Read the model definition and answer for the solid it produces. Units are mm, in the model's axes. Coordinates: 2 decimals unless noted, no trailing zeros. Loops run counter-clockwise (first coordinate to the right, second up) from the corner with the lowest first, then second, coordinate; pieces in that order, holes last.
Q1. Section C-C (x = -10.5) is taken. Give the vertices of the cut face in (y, z).
Q2. Section B-B (y = 23.5) is taken. Give the vertices of the cut face in (x, z), then the cut area to 3 significant figures.
Q3. Straight lines are drawn through the part: line 1 (Y direction, x = -3, z = -0.3); line 2 (X direction, y = 18.5, z = -0.4); line 3 (X direction, y = 9.5, z = -0.95). For each, find the intervals that lie inside material, in ascending order.
Q4. A flat-ended cylindrical pin translates along its axis: P1, Ø0.6, axis at x = -15, z = -0.5, coming from the +Y side. Find the tip coordinate at first contact, or state that the pin passes through.
Q5. Section A-A (z = -1) is taken. Give the vertices of the cut face in (x, y).
from build123d import *

# Parameters (mm, degrees)
SM_BASE_FLANGE_1_DEPTH = 1.2


# Sheet-metal steps are written as plain solids
with BuildPart() as part:
    # Sketch 1 → 基体-法兰1 (new body)
    with BuildSketch(Plane.XY):
        with BuildLine():
            Line((0, 0), (-26, 0))
            ThreePointArc((-26, 0), (-29, 3), (-26, 6))
            ThreePointArc((-26, 6), (-23, 9), (-26, 12))
            ThreePointArc((-26, 12), (-29, 15), (-26, 18))
            Line((-26, 18), (0, 18))
            Line((0, 18), (11.606526016, 25.828700649))
            ThreePointArc((11.606526016, 25.828700649), (15.771217444, 25.019166641), (14.961683437, 20.854475213))
            ThreePointArc((14.961683437, 20.854475213), (14.152149429, 16.689783785), (18.316840857, 15.880249778))
            ThreePointArc((18.316840857, 15.880249778), (22.481532285, 15.070715771), (21.671998278, 10.906024343))
            Line((21.671998278, 10.906024343), (5.503152266, 0))
            Line((5.503152266, 0), (0, 0))
        make_face()
    extrude(amount=-SM_BASE_FLANGE_1_DEPTH)


solid = part.part
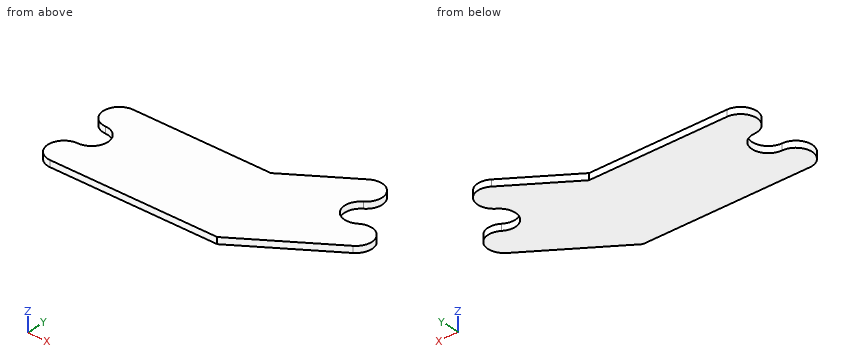
Numbers:
1. outline: (0, -1.2) - (18, -1.2) - (18, 0) - (0, 0) - close
2. outline: (8.15, -1.2) - (16.28, -1.2) - (16.28, 0) - (8.15, 0) - close
2. area: 9.75 mm2
3. line 1: y = 0 to 18
3. line 2: x = 0.74 to 13.64
3. line 3: x = -23.04 to 19.59
4. P1: stops at y = 18
5. outline: (-26, 0) - (5.5, 0) - (21.67, 10.91) arc R3 ccw to (18.32, 15.88) arc R3 cw to (14.96, 20.85) arc R3 ccw to (11.61, 25.83) - (0, 18) - (-26, 18) arc R3 ccw to (-26, 12) arc R3 cw to (-26, 6) arc R3 ccw to start
